Print and shaded views of the part. All mm, measured from the part's lowest x, y and z. Round coordinates to 2 decimals unless told otherwise and drop trailing zeros. Order: outer loops, then holes, each group sorted by start corner. A loop starts at its lowest first (then second) coordinate and runs counter-clockwise, first axis right, second up. Notation, with made-up numbers: (-34.75, -6.5) - (20.25, -6.5) arc R15 cw to (20.25, 12.5) - close; hole circle Ø3 at (26.25, -24). An arc over 180 degrees is marked (long way). Return JSON: item names as keys, results as strings. Group by question number.
Item 1: Two-plate mould, pull along X, no slides. Class the marked faces 1, 2, 3 and 4: released by +X, released by -X, zero draft, split by the parting line, or undercut.
Item 2: Saw through at C-C on y = 22. List the corners of the cut face in (x, z).
Item 3: Saw through at D-D on y = 18.5. List the corners of the cut face in (x, z).
Item 4: Saw through at B-B on z = 7. List the corners of the cut face in (x, y), and give its area (3 significant figures).
Item 5: Probe probe 1 along Y at (x, z) = (22.5, 1.1); probe 2 along X at (y, z) = (23.25, 13.5); probe 3 along X at (y, z) = (22.25, 0.5). List the from-to ranges inside material, lowest first.
Item 6: Drop flat-ended pins along their axis: pin 1 (4 mm diameter, centred on y = 19, z = 3.5, fed in from +X); pin 2 (3 mm diameter, centred on y = 5, z = 6, fed in from -X); pin 3 (6 mm diameter, centred on x = 14.5, y = 4.5, fed in from -Z); pin 4 (7.5 mm diameter, centred on x = 26, y = 13.5, fed in from +Z). Give the stop position or say it passes through.
Item 7: Saw through at A-A on x = 22.5. List the corners of the cut face in (y, z).
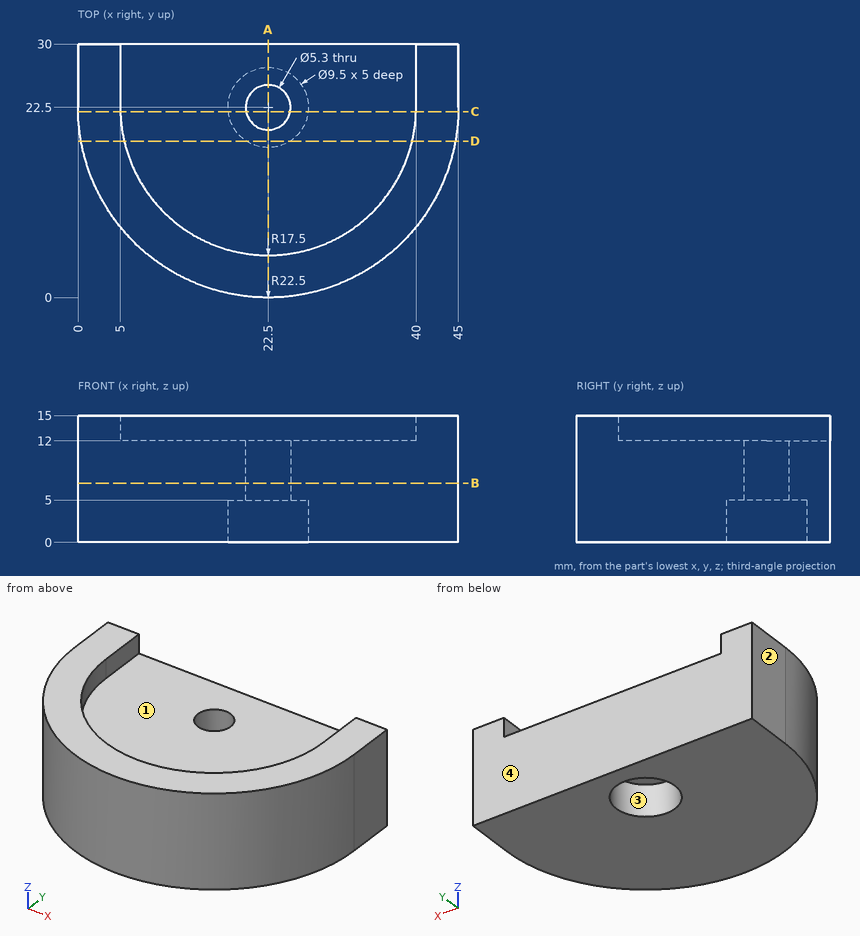
Filled in:
{
 "1": {"face 1": "undercut", "face 2": "released by -X", "face 3": "undercut", "face 4": "zero draft"},
 "2": {"outline": "(0.01, 0) - (17.78, 0) - (17.78, 5) - (19.9, 5) - (19.9, 12) - (5.01, 12) - (5.01, 15) - (0.01, 15) - close; (25.1, 5) - (27.22, 5) - (27.22, 0) - (44.99, 0) - (44.99, 15) - (39.99, 15) - (39.99, 12) - (25.1, 12) - close"},
 "3": {"outline": "(0.36, 0) - (19.94, 0) - (19.94, 5) - (25.06, 5) - (25.06, 0) - (44.64, 0) - (44.64, 15) - (39.54, 15) - (39.54, 12) - (5.46, 12) - (5.46, 15) - (0.36, 15) - close"},
 "4": {"outline": "(0, 22.5) arc R22.5 ccw to (45, 22.5) - (45, 30) - (0, 30) - close; hole circle Ø5.3 at (22.5, 22.5)", "area": "1,110 mm^2"},
 "5": {"probe 1": "y = 0 to 17.75, 27.25 to 30", "probe 2": "x = 0 to 5, 40 to 45", "probe 3": "x = 0 to 17.76, 27.24 to 45"},
 "6": {"pin 1": "stops at x = 44.95", "pin 2": "stops at x = 6.68", "pin 3": "stops at z = 0", "pin 4": "stops at z = 12"},
 "7": {"outline": "(0, 0) - (17.75, 0) - (17.75, 5) - (19.85, 5) - (19.85, 12) - (5, 12) - (5, 15) - (0, 15) - close; (25.15, 5) - (27.25, 5) - (27.25, 0) - (30, 0) - (30, 12) - (25.15, 12) - close"}
}
